Geometry: final body of the model. Coordinates: model frame, mm. Give positions to 0.01 mm unless a question says otherwise; leave off trailing zeros. Write each loop counter-clockwise with the first axis right and the second up, starting at its lowest first coordinate (ties: lowest second). Pieces come first, ordered by that corner, then holes. Notation, with made-up numbers: M 74,67 L 83,67 A30 ccw 83,92 Z; hole C 41,-1.5 d10. An arc over 180 degrees is marked long. Answer as a JSON object with one key per item and string values.
from build123d import *

# Parameters (mm, degrees)
F0_R       = 11.15
F0_R_2     = 9.15
F1_DEPTH   = 7.5
F2_SIZE2   = 1.5
F2_SIZE    = 1
F2_2_SIZE2 = 1.5
F2_2_SIZE  = 1
F3_R       = 0.2


# Not quite as in the source:
# - a feature names something its author has since deleted; it is built from what else it names


with BuildPart() as f1:
    # F0 (on Top) → F1 (new body)
    with BuildSketch(Plane.XY):
        Circle(F0_R)
        Circle(F0_R_2, mode=Mode.SUBTRACT)
    extrude(amount=F1_DEPTH)

    # F2
    f2_edges = [f1.edges().sort_by_distance(p)[0] for p in [
        (-11.15, 0, 7.5),
    ]]
    f2_side = f1.faces().sort_by_distance((-10.83463, 0, 7.5))[0]
    chamfer(f2_edges, length=F2_SIZE, length2=F2_SIZE2, reference=f2_side)

    # F2#2
    f2_2_edges = [f1.edges().sort_by_distance(p)[0] for p in [
        (-11.15, 0, 0),
    ]]
    f2_2_side = f1.faces().sort_by_distance((-10.83463, 0, 0))[0]
    chamfer(f2_2_edges, length=F2_2_SIZE, length2=F2_2_SIZE2, reference=f2_2_side)

    # F3
    f3_edges = [f1.edges().sort_by_distance(p)[0] for p in [
        (-9.15, 0, 7.5),
    ]]
    fillet(f3_edges, radius=F3_R)


solid = f1.part
1) Pull-direction query (Y, two-part tool) for faces 1 (the cylindrical face through (4.919, 7.715, 3.599)), 2 (the cylindrical face through (10.635, 3.349, 3.718)), 3 (the flat face through (-5, 8, 0)); classes: pulls with the +Y half, pulls with the -Y half, needs draft (parallel to the pull), parting line crosses it, or undercut.
Geometry check:
{"face 1": "undercut", "face 2": "parting line crosses it", "face 3": "needs draft"}
2) Cut plane A-A on x = 0. Return loops of the section in (y, z), and give its area (3 significant figures).
Geometry check:
{"outline": "M -11.15,1.5 L -10.15,0 L -9.15,0 L -9.15,7.3 A0.2 ccw -9.35,7.5 L -10.15,7.5 L -11.15,6 Z; M 9.15,0 L 10.15,0 L 11.15,1.5 L 11.15,6 L 10.15,7.5 L 9.35,7.5 A0.2 ccw 9.15,7.3 Z", "area": "27.0 mm2"}
3) Line query: line 1 (Y direction, x = 0, z = 4.5); line 2 (X direction, y = -7.25, z = 3.75); line 3 (Y direction, x = 0, z = 6.25). Output: solid intervals per line, ascending. Write a range as from..to.
Geometry check:
{"line 1": "y = -11.15..-9.15, 9.15..11.15", "line 2": "x = -8.47..-5.58, 5.58..8.47", "line 3": "y = -10.98..-9.15, 9.15..10.98"}
4) Contact query for flat-ended pins moving along their axis: P1, Ø1, axis at x = 7.5, z = 2.5, coming from the -Y side; P2, Ø3, axis at y = 5, z = 3, coming from the -X side. Output: stop coordinate, or through.
Geometry check:
{"P1": "stops at y = -8.68", "P2": "stops at x = -10.59"}
5) Cut plane C-C on z = 2.5. Return loops of the section in (x, y).
Geometry check:
{"outline": "C 0,0 d22.3; hole C 0,0 d18.3"}
